```python
from build123d import *

# Parameters (mm, degrees)
BOSS_EXTRU_1_DEPTH         = 6.5
ESQUISSE2_W                = 18
ESQUISSE2_H                = 53.786822236
ENL_V_MAT_EXTRU_1_DEPTH    = 6.5
D_GAGEMENT_M61_D           = 6.6
R_P_TITION_LIN_AIRE1_COUNT = 7
R_P_TITION_LIN_AIRE1_PITCH = 60


with BuildPart() as part:
    # Esquisse1 → Boss.-Extru.1 (new body)
    with BuildSketch(Plane.XY):
        Polygon((416, -265.000000009), (416, -251.75), (456, -251.75), (456, 251.75), (-456, 251.75), (-456, -251.75), (-416, -251.75), (-416, -261.75000001), (-397.670089581, -261.75000001), (-397.670089581, -281.75000001), (-416, -281.75000001), (-416, -291.75), (416, -291.75), (416, -288.5), (416, -285.000000009), (397.67, -285.000000009), (397.67, -265.000000009), align=None)
    extrude(amount=BOSS_EXTRU_1_DEPTH)

    # Esquisse2 → Enl_v. mat.-Extru.1 (cut)
    with BuildSketch(Plane.XY.offset(6.5)):
        with Locations((-436.999999996, 218.356588882)):
            Rectangle(ESQUISSE2_W, ESQUISSE2_H)
    enl_v_mat_extru_1 = extrude(amount=-ENL_V_MAT_EXTRU_1_DEPTH, mode=Mode.SUBTRACT)

    # Sym_trie1: Enl_v. mat.-Extru.1 across plane
    add(enl_v_mat_extru_1.mirror(Plane(origin=(0, 0, 0), x_dir=(0, 0, 1), z_dir=(1, 0, 0))), mode=Mode.SUBTRACT)

    # D_gagement M61 (through all)
    with Locations(Plane(origin=(0, 0, 0), x_dir=(-1, 0, 0), z_dir=(0, 0, -1))):
        with Locations((436.025271582, 166.031516539)):
            Hole(D_GAGEMENT_M61_D / 2)

    # Esquisse5 → Chambrage pour vis _ t_te ronde bomb_e M (revolve, cut)
    with BuildSketch(Plane(origin=(-436.025271582, 166.031516539, 6.5), x_dir=(0, -1, 0), z_dir=(1, 0, 0))):
        Polygon((0, 0), (0, 6.5), (3.3, 6.5), (3.3, 4.625), (3.325, 4.6), (6.5, 4.6), (6.5, 0), align=None)
    chambrage_pour_vis_t_te_ronde_bomb_e_m = revolve(axis=Axis((-436.025271582, 166.031516539, 12.85), (0, 0, -1)), mode=Mode.SUBTRACT)

    # R_p_tition lin_aire1: Chambrage pour vis _ t_te ronde bomb_e M ×7
    with Locations(*[(0, -i * R_P_TITION_LIN_AIRE1_PITCH, 0) for i in range(1, R_P_TITION_LIN_AIRE1_COUNT)]):
        add(chambrage_pour_vis_t_te_ronde_bomb_e_m, mode=Mode.SUBTRACT)

    # Sym_trie2: Chambrage pour vis _ t_te ronde bomb_e M across plane
    add(chambrage_pour_vis_t_te_ronde_bomb_e_m.mirror(Plane(origin=(0, 0, 0), x_dir=(0, 0, 1), z_dir=(1, 0, 0))), mode=Mode.SUBTRACT)

    # Sym_trie2 copy 1 sketch → Sym_trie2 copy 1 (revolve, cut)
    with BuildSketch(Plane(origin=(436.025271582, 106.031516539, 6.5), x_dir=(0, -1, 0), z_dir=(-1, 0, 0))):
        Polygon((0, 0), (0, -6.5), (3.3, -6.5), (3.3, -4.625), (3.325, -4.6), (6.5, -4.6), (6.5, 0), align=None)
    revolve(axis=Axis((436.025271582, 106.031516539, 12.85), (0, 0, 1)), mode=Mode.SUBTRACT)

    # Sym_trie2 copy 2 sketch → Sym_trie2 copy 2 (revolve, cut)
    with BuildSketch(Plane(origin=(436.025271582, 46.031516539, 6.5), x_dir=(0, -1, 0), z_dir=(-1, 0, 0))):
        Polygon((0, 0), (0, -6.5), (3.3, -6.5), (3.3, -4.625), (3.325, -4.6), (6.5, -4.6), (6.5, 0), align=None)
    revolve(axis=Axis((436.025271582, 46.031516539, 12.85), (0, 0, 1)), mode=Mode.SUBTRACT)

    # Sym_trie2 copy 3 sketch → Sym_trie2 copy 3 (revolve, cut)
    with BuildSketch(Plane(origin=(436.025271582, -13.968483461, 6.5), x_dir=(0, -1, 0), z_dir=(-1, 0, 0))):
        Polygon((0, 0), (0, -6.5), (3.3, -6.5), (3.3, -4.625), (3.325, -4.6), (6.5, -4.6), (6.5, 0), align=None)
    revolve(axis=Axis((436.025271582, -13.968483461, 12.85), (0, 0, 1)), mode=Mode.SUBTRACT)

    # Sym_trie2 copy 4 sketch → Sym_trie2 copy 4 (revolve, cut)
    with BuildSketch(Plane(origin=(436.025271582, -73.968483461, 6.5), x_dir=(0, -1, 0), z_dir=(-1, 0, 0))):
        Polygon((0, 0), (0, -6.5), (3.3, -6.5), (3.3, -4.625), (3.325, -4.6), (6.5, -4.6), (6.5, 0), align=None)
    revolve(axis=Axis((436.025271582, -73.968483461, 12.85), (0, 0, 1)), mode=Mode.SUBTRACT)

    # Sym_trie2 copy 5 sketch → Sym_trie2 copy 5 (revolve, cut)
    with BuildSketch(Plane(origin=(436.025271582, -133.968483461, 6.5), x_dir=(0, -1, 0), z_dir=(-1, 0, 0))):
        Polygon((0, 0), (0, -6.5), (3.3, -6.5), (3.3, -4.625), (3.325, -4.6), (6.5, -4.6), (6.5, 0), align=None)
    revolve(axis=Axis((436.025271582, -133.968483461, 12.85), (0, 0, 1)), mode=Mode.SUBTRACT)

    # Sym_trie2 copy 6 sketch → Sym_trie2 copy 6 (revolve, cut)
    with BuildSketch(Plane(origin=(436.025271582, -193.968483461, 6.5), x_dir=(0, -1, 0), z_dir=(-1, 0, 0))):
        Polygon((0, 0), (0, -6.5), (3.3, -6.5), (3.3, -4.625), (3.325, -4.6), (6.5, -4.6), (6.5, 0), align=None)
    revolve(axis=Axis((436.025271582, -193.968483461, 12.85), (0, 0, 1)), mode=Mode.SUBTRACT)


solid = part.part
```
Design review of the part built by this model. Coordinates are the model's own, in mm. Coordinates: 2 decimals unless noted, no trailing zeros. Loops run counter-clockwise (first coordinate to the right, second up) from the corner with the lowest first, then second, coordinate; pieces in that order, holes last. Notation, with made-up numbers: (49, -9) - (53, -9) arc R20 cw to (53, 24) - close; hole circle Ø3 at (74.5, 71.5). An arc over 180 degrees is marked (long way). Use CSV: the item, a comma, the result in double quotes. Start each with the question number.
1) Wall thickness on L1, parallel to X at y = 164.5, z = 1.25: over which ranges is the line inside the solid? List them lowest first. Write a range as from..to.
2) Consider section A-A on y = 207. Write out the cut boundary in (x, z).
3) Consider section B-B on z = 4. Give the number of separate pieces and of enclosed holes in the cut face, then the cut area to 3 significant figures.
4) For pin 1 Ø2 at (y, z) = (-261, 3.5) entering from +X; pin 2 Ø3 at (y, z) = (-286.5, 3.5) entering from -X; pin 3 Ø10.5 at (x, y) = (-436.03, -193.97) entering from +Z, all flat-tipped, find the tip position at first contact; note any pin that passes through.
Geometry says:
1,L1,"-456..-438.95, -433.1..433.1, 438.95..456"
2,outline,"(-456, 0) - (-446, 0) - (-446, 6.5) - (-456, 6.5) - close; (-428, 0) - (428, 0) - (428, 6.5) - (-428, 6.5) - close; (446, 0) - (456, 0) - (456, 6.5) - (446, 6.5) - close"
3,separate pieces,"1"
3,enclosed holes,"16"
3,area,"488,000 mm^2"
4,pin 1,"x = 416"
4,pin 2,"x = -416"
4,pin 3,"z = 1.9"
